```python
from build123d import *

# Parameters (mm, degrees)
F0_W     = 60
F0_H     = 80
F1_DEPTH = 25
F2_R     = 12.5
F2_R_2   = 7.5
F3_DEPTH = 50


with BuildPart() as f1:
    # F0 (on Front) → F1 (new body, symmetric)
    with BuildSketch(Plane.XZ):
        Rectangle(F0_W, F0_H)
    extrude(amount=F1_DEPTH, both=True)

    # F2 (on face) → F3 (cut, through all)
    with BuildSketch(Plane.XZ.offset(25)):
        with Locations((-10, 20)):
            Circle(F2_R)
        with Locations((5, -16)):
            Circle(F2_R_2)
    extrude(amount=-F3_DEPTH, mode=Mode.SUBTRACT)


solid = f1.part
```
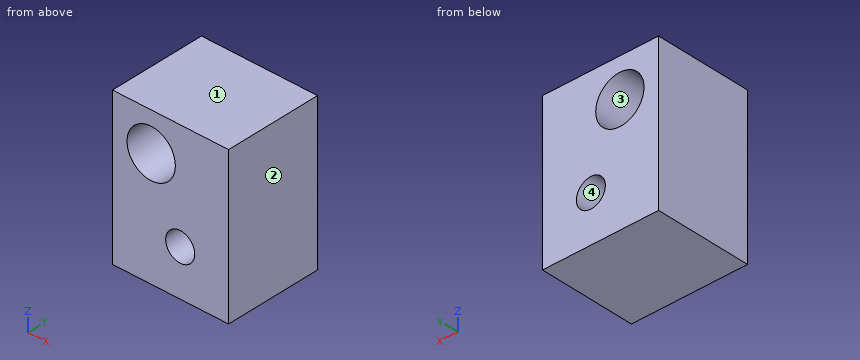
Model file for the job. Use its own axes, mm. Face numbers are marked on the shaded views. Coordinates: 2 decimals unless noted, no trailing zeros. Order: outer loops, then holes, each group sorted by start corner. A loop starts at its lowest first (then second) coordinate and runs counter-clockwise, first axis right, second up. Notation, with made-up numbers: (17.25, 80.5) -> (64.25, 80.5) arc R10 cw to (64.25, 93.5) -> close; hole circle Ø3 at (-10.75, -28.75). An arc over 180 degrees is marked (long way). Return JSON: item names as keys, results as strings.
Item 1: Wall check: line 1 along Z through (x, y) = (4.5, 15.5); line 2 along Z through (x, y) = (-10, -5); line 3 along X through (y, z) = (-13, 28.5). Give the ranges that are in metal, low to high. Write a range as from..to.
Model answer:
{"line 1": "z = -40..-23.48, -8.52..40", "line 2": "z = -40..7.5, 32.5..40", "line 3": "x = -30..-19.17, -0.83..30"}
Item 2: Mould opens along Z. For the marked faces 1, 2, 3 and 4 say: pulls with the +Z half, pulls with the -Z half, needs draft (parallel to the pull), parting line crosses it, or undercut.
Model answer:
{"face 1": "pulls with the +Z half", "face 2": "needs draft", "face 3": "undercut", "face 4": "undercut"}
Item 3: Pin check, flat tip, straight feed: P1, Ø17, axis at x = 5, z = -16, coming from the +Y side. Stop position of the tip, or through.
Model answer:
{"P1": "stops at y = 25"}
Item 4: Slice it at C-C (y = 5.5). Write the cut outline in (x, z), then the cut area to 3 significant figures.
Model answer:
{"outline": "(-30, -40) -> (30, -40) -> (30, 40) -> (-30, 40) -> close; hole circle Ø25 at (-10, 20); hole circle Ø15 at (5, -16)", "area": "4,130 mm²"}
Item 5: Slice it at B-B (x = 5). Write the cut outline in (y, z), then the cut area to 3 significant figures.
Model answer:
{"outline": "(-25, -40) -> (25, -40) -> (25, -23.5) -> (-25, -23.5) -> close; (-25, -8.5) -> (25, -8.5) -> (25, 40) -> (-25, 40) -> close", "area": "3,250 mm²"}
Item 6: Slice it at A-A (z = -16). Write the cut outline in (x, y).
Model answer:
{"outline": "(-30, -25) -> (-2.5, -25) -> (-2.5, 25) -> (-30, 25) -> close; (12.5, -25) -> (30, -25) -> (30, 25) -> (12.5, 25) -> close"}
